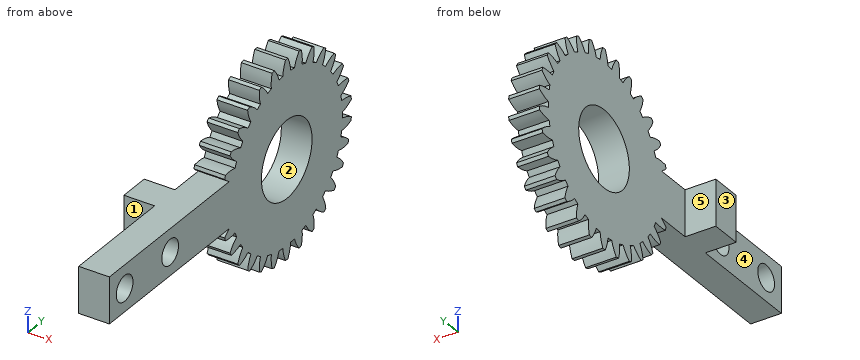
```python
from build123d import *

# Parameters (mm, degrees)
BASPROSKE_W         = 4
BASPROSKE_H         = 12.8
TOOTHCUT_DEPTH      = 19.538608362
TEETHCUTS_COUNT     = 30
TEETHCUTS_ANGLE     = 348
BORSKE_R            = 5
BORE_DEPTH          = 50.0000508
SKETCH_1_W          = 6
SKETCH_1_H          = 28.363297546
EXTRUDE_1_DEPTH     = 4
SKETCH_4_W          = 2
SKETCH_4_H          = 15
CUT_EXTRUDE_2_DEPTH = 6
SKETCH_6_R          = 1.65
CUT_EXTRUDE_3_DEPTH = 4
EXTRUDE_START       = 2
SKETCH_8_W          = 6
SKETCH_8_H          = 15
SKETCH_8_R          = 1.65
EXTRUDE_2_DEPTH     = 2
SKETCH_9_W          = 4
SKETCH_9_H          = 4
EXTRUDE_3_DEPTH     = 6


with BuildPart() as part:
    # BasProSke → Base-Revolve (revolve)
    with BuildSketch(Plane(origin=(0, 0, 0), x_dir=(1, 0, 0), z_dir=(0, 1, 0)), mode=Mode.PRIVATE) as base_revolve_sk:
        with Locations((2, 6.4)):
            Rectangle(BASPROSKE_W, BASPROSKE_H)
    revolve(base_revolve_sk.sketch.rotate(Axis((-10, 0, 0), (1, 0, 0)), 180), axis=Axis((-10, 0, 0), (1, 0, 0)))

    # TooCutSke → ToothCut (cut, through all)
    with BuildSketch(Plane(origin=(0, 0, 0), x_dir=(0, 0, -1), z_dir=(1, 0, 0))):
        with BuildLine():
            ThreePointArc((0.37243947, 10.992692566), (0, 10.999), (-0.37243947, 10.992692566))
            ThreePointArc((-0.37243947, 10.992692566), (-0.655704499, 11.922595954), (-1.120515575, 12.776358245))
            ThreePointArc((-1.120515575, 12.776358245), (0, 12.8254), (1.120515575, 12.776358245))
            ThreePointArc((1.120515575, 12.776358245), (0.655704499, 11.922595954), (0.37243947, 10.992692566))
        make_face()
    toothcut = extrude(amount=TOOTHCUT_DEPTH, mode=Mode.SUBTRACT)

    # TeethCuts: ToothCut ×30 about axis
    teethcuts_axis = Axis((-10, 0, 0), (1, 0, 0))
    for i in range(1, TEETHCUTS_COUNT):
        add(toothcut.rotate(teethcuts_axis, i * TEETHCUTS_ANGLE / (TEETHCUTS_COUNT - 1)), mode=Mode.SUBTRACT)

    # BorSke → Bore (cut, symmetric)
    with BuildSketch(Plane(origin=(0, 0, 0), x_dir=(0, 0, -1), z_dir=(1, 0, 0))):
        with Locations(Location((0, 0, 0), (0, 0, 180))):
            Circle(BORSKE_R)
    extrude(amount=BORE_DEPTH, both=True, mode=Mode.SUBTRACT)

    # 草图1 → 凸台-拉伸1 (add)
    with BuildSketch(Plane(origin=(4, 0, 0), x_dir=(0, 0, -1), z_dir=(1, 0, 0))):
        with Locations((0, -20.818351227)):
            Rectangle(SKETCH_1_W, SKETCH_1_H)
    extrude(amount=-EXTRUDE_1_DEPTH)

    # 草图4 → 切除-拉伸2 (cut)
    with BuildSketch(Plane(origin=(0, 0, -3), x_dir=(-1, 0, 0), z_dir=(0, 0, -1))):
        with Locations((-1, -27.5)):
            Rectangle(SKETCH_4_W, SKETCH_4_H)
    extrude(amount=-CUT_EXTRUDE_2_DEPTH, mode=Mode.SUBTRACT)

    # 草图6 → 切除-拉伸3 (cut)
    with BuildSketch(Plane.ZY.offset(-2)):
        with Locations((0, -23)):
            Circle(SKETCH_6_R)
        with Locations((0, -32)):
            Circle(SKETCH_6_R)
    extrude(amount=-CUT_EXTRUDE_3_DEPTH, mode=Mode.SUBTRACT)

    # 草图8 → 凸台-拉伸2 (add)
    with BuildSketch(Plane.ZY.offset(-2).offset(EXTRUDE_START)):
        with Locations((0, -27.5)):
            Rectangle(SKETCH_8_W, SKETCH_8_H)
        with Locations((0, -23)):
            Circle(SKETCH_8_R, mode=Mode.SUBTRACT)
        with Locations((0, -32)):
            Circle(SKETCH_8_R, mode=Mode.SUBTRACT)
    extrude(amount=-EXTRUDE_2_DEPTH)

    # 草图9 → 凸台-拉伸3 (add)
    with BuildSketch(Plane.XY.offset(3)):
        with Locations((-2, -18)):
            Rectangle(SKETCH_9_W, SKETCH_9_H)
    extrude(amount=-EXTRUDE_3_DEPTH)


solid = part.part
```
Check sheet for the modelled part. Datum: model origin and axes. Units: mm. Face numbers are marked on the shaded views. A direction names the side the tool comes from. Round coordinates to 2 decimals unless told otherwise and drop trailing zeros. Order: outer loops, then holes, each group sorted by start corner. A loop starts at its lowest first (then second) coordinate and runs counter-clockwise, first axis right, second up. Notation, with made-up numbers: M 4.5,40 L 11.5,40 A15 ccw 11.5,57 Z; hole C 67,25.5 d10. An arc over 180 degrees is marked long. Answer in a Markdown table with one row per item.
(1) Section check A-A on y = -32. Record the boundary of the cut face in (x, z), plus the area to 3 significant figures.
Findings:
| item | result |
|---|---|
| outline | M 0,-3 L 4,-3 L 4,-1.65 L 0,-1.65 Z; M 0,1.65 L 4,1.65 L 4,3 L 0,3 Z |
| area | 10.8 mm^2 |
(2) Gauge pin test, flat ends, axial feed: pin 1 (1.2 mm diameter, centred on x = -2, z = 0, fed in from -Y); pin 2 (7.5 mm diameter, centred on y = -5.5, z = 3.5, fed in from -X); pin 3 (4 mm diameter, centred on x = 3, y = -19, fed in from +Z). Record the tip position at first contact, or that the pin passes through.
Findings:
| item | result |
|---|---|
| pin 1 | stops at y = -20 |
| pin 2 | stops at x = 0 |
| pin 3 | stops at z = 3 |
(3) Draft check along Z on the marked faces 1 and 2. Enter one of: +Z half, -Z half, draft (parallel to the pull), parting line (faces both ways), or undercut.
Findings:
| item | result |
|---|---|
| face 1 | draft |
| face 2 | undercut |
(4) Set-up check for the marked faces 3, 4 and 5: record each of +Z, -Z, +X, -X, +Y, -Y from which the full face is reachable in a straight line by a thin tool's end or side.
Findings:
| item | result |
|---|---|
| face 3 | +Z, -Z, -X, +Y, -Y |
| face 4 | +Z, -Z, -X, -Y |
| face 5 | +Z, -Z, -X, +Y |
(5) Section check C-C on y = -26. Record the boundary of the cut face in (x, z), plus the area to 3 significant figures.
Findings:
| item | result |
|---|---|
| outline | M 0,-3 L 4,-3 L 4,3 L 0,3 Z |
| area | 24.0 mm^2 |
(6) Material ranges on line 1 along Y through (x, z) = (3.15, 0); line 2 along Z through (x, y) = (1.5, -12); line 3 along X through (y, z) = (-11.5, -2.25), recorded low to high. Write a range as from..to.
Findings:
| item | result |
|---|---|
| line 1 | y = -35..-33.65, -30.35..-24.65, -21.35..-5, 5..11 |
| line 2 | z = -4.19..-3.5, -3..3, 3.5..4.19 |
| line 3 | x = 0..4 |
(7) Section check D-D on x = -2. Record the boundary of the cut face in (y, z).
Findings:
| item | result |
|---|---|
| outline | M -20,-3 L -16,-3 L -16,3 L -20,3 Z |
(8) Section check B-B on x = 3.25. Give the number of separate pieces and of enclosed holes in the cut face, plus the area to 3 significant figures.
Findings:
| item | result |
|---|---|
| separate pieces | 1 |
| enclosed holes | 3 |
| area | 487 mm^2 |
